```python
from build123d import *

# Parameters (mm, degrees)
F1_DEPTH  = 25.4
F0_W      = 9.8233733336
F0_H      = 1.6087094842
F2_DEPTH  = 31.75
F0_H_2    = 9.4561445239
F3_DEPTH  = 19.05
F5_DEPTH  = 4.318
F8_R      = 4.125
F9_DEPTH  = 7
F11_R     = 4.125
F7_R      = 4.125
F12_DEPTH = 15.24
F6_R      = 4.125
F10_R     = 4.125
F13_DEPTH = 15.24
F14_DEPTH = 6.35
F15_DEPTH = 6.35


with BuildPart() as f1:
    # F0 (on Front) → F1 (new body, symmetric)
    with BuildSketch(Plane.XZ):
        Polygon((38.1, 9.4561445239), (-35.3728867915, 9.4561445239), (-38.1, 7.3570762504), (-38.1, 1.6087094842), (-28.2766266664, 1.6087094842), (-28.2766266664, 0), (-28.2766266664, -9.4561445239), (28.2766266664, -9.4561445239), (28.2766266664, 0), (28.2766266664, 1.6087094842), (38.1, 1.6087094842), align=None)
    extrude(amount=F1_DEPTH, both=True)

    # F0 (on Front) → F2 (join, symmetric)
    with BuildSketch(Plane.XZ):
        with Locations((-33.1883133332, 0.8043547421)):
            Rectangle(F0_W, F0_H)
        with Locations((33.1883133332, 0.8043547421)):
            Rectangle(F0_W, F0_H)
    extrude(amount=F2_DEPTH, both=True)

    # F0 (on Front) → F3 (join, symmetric)
    with BuildSketch(Plane.XZ):
        with Locations((-33.1883133332, -4.728072262)):
            Rectangle(F0_W, F0_H_2)
        with Locations((33.1883133332, -4.728072262)):
            Rectangle(F0_W, F0_H_2)
    extrude(amount=F3_DEPTH, both=True)

    # F4 (on face) → F5 (join)
    with BuildSketch(Plane(origin=(-38.1, 0, 0), x_dir=(0, -1, 0), z_dir=(-1, 0, 0))):
        Polygon((-19.05, 0), (19.05, 0), (25.4, 0), (25.4, 1.6087094842), (25.4, 7.3570762504), (-25.4, 7.3570762504), (-25.4, 1.6087094842), (-25.4, 0), align=None)
    extrude(amount=F5_DEPTH)

    # F8 (on face) → F9 (join)
    with BuildSketch(Plane.XY.offset(9.4561445239)):
        Circle(F8_R)
    extrude(amount=F9_DEPTH)

    # F11 (on face) + F7 (on face) → F12 (join)
    with BuildSketch(Plane(origin=(0, 19.05, 0), x_dir=(-1, 0, 0), z_dir=(0, 1, 0))):
        with Locations((-33.721, -5.0771445239)):
            Circle(F11_R)
    with BuildSketch(Plane(origin=(0, 19.05, 0), x_dir=(-1, 0, 0), z_dir=(0, 1, 0))):
        with Locations((33.721, -5.0771445239)):
            Circle(F7_R)
    extrude(amount=F12_DEPTH)

    # F6 (on face) + F10 (on face) → F13 (join)
    with BuildSketch(Plane.XZ.offset(19.05)):
        with Locations((-33.721, -5.0771445239)):
            Circle(F6_R)
    with BuildSketch(Plane.XZ.offset(19.05)):
        with Locations((33.721, -5.0771445239)):
            Circle(F10_R)
    extrude(amount=F13_DEPTH)

    # F14 (add): faces of the model
    f14_faces = [f1.faces().sort_by_distance(p)[0] for p in [
        (-33.1883133332, -19.05, -0.1363515064),
        (33.1883133332, -19.05, -9.3197930175),
    ]]
    extrude(f14_faces, amount=F14_DEPTH)

    # F15 (add): faces of the model
    f15_faces = [f1.faces().sort_by_distance(p)[0] for p in [
        (33.1883133332, 19.05, -9.3197930175),
        (-33.1883133332, 19.05, -0.1363515064),
    ]]
    extrude(f15_faces, amount=F15_DEPTH)


solid = f1.part
```
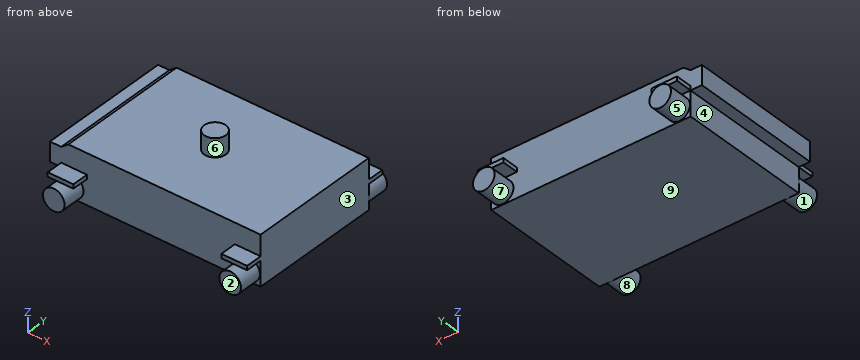
Verification items for the finished model (mm, model axes). Face numbers are marked on the shaded views. A direction names the side the tool comes from. Round coordinates to 2 decimals unless told otherwise and drop trailing zeros. Loops run counter-clockwise (first coordinate to the right, second up) from the corner with the lowest first, then second, coordinate; pieces in that order, holes last. Notation, with made-up numbers: (50, 86.5) -> (105, 86.5) arc R12 ccw to (105, 109.5) -> close; hole circle Ø3 at (43.25, 32). An arc over 180 degrees is marked (long way). Answer as a JSON object with one key per item and string values.
Q1. Section check C-C (z = -2.5). Record the boundary of the cut face in (x, y).
Data:
{"outline": "(-38.1, -25.4) -> (-36.94, -25.4) -> (-36.94, -34.29) -> (-30.5, -34.29) -> (-30.5, -25.4) -> (30.5, -25.4) -> (30.5, -34.29) -> (36.94, -34.29) -> (36.94, -25.4) -> (38.1, -25.4) -> (38.1, 25.4) -> (36.94, 25.4) -> (36.94, 34.29) -> (30.5, 34.29) -> (30.5, 25.4) -> (-30.5, 25.4) -> (-30.5, 34.29) -> (-36.94, 34.29) -> (-36.94, 25.4) -> (-38.1, 25.4) -> close"}
Q2. Scan lines: line 1 (Z direction, x = -24, y = -10.5); line 2 (Y direction, x = 32, z = 0.5); line 3 (Y direction, x = 8.5, z = -4.75). Record each from-to range of solid material in increasing order. Write a range as from..to.
Data:
{"line 1": "z = -9.46..9.46", "line 2": "y = -31.75..31.75", "line 3": "y = -25.4..25.4"}
Q3. Section check D-D (x = 9.5). Record the boundary of the cut face in (y, z), then the cut area to 3 significant figures.
Data:
{"outline": "(-25.4, -9.46) -> (25.4, -9.46) -> (25.4, 9.46) -> (-25.4, 9.46) -> close", "area": "961 mm2"}
Q4. Access from +Z, -Z, +X, -X, +Y, -Y to the whole of each face (thin tool, end or side, straight path). Record for the marked faces 1, 2, 3, 4 and 5.
Data:
{"face 1": "-Y", "face 2": "+Z, -Z, +X, -X, -Y", "face 3": "+Z, -Z, +X, +Y, -Y", "face 4": "-Z, -X, +Y, -Y", "face 5": "+Y"}
Q5. Section check A-A (x = 0). Record the boundary of the cut face in (y, z) (3 decimals), then the cut area to 3 significant figures.
Data:
{"outline": "(-25.4, -9.456) -> (25.4, -9.456) -> (25.4, 9.456) -> (4.125, 9.456) -> (4.125, 16.456) -> (-4.125, 16.456) -> (-4.125, 9.456) -> (-25.4, 9.456) -> close", "area": "1,020 mm2"}
Q6. Section check B-B (y = 15.5). Record the boundary of the cut face in (x, z).
Data:
{"outline": "(-42.42, 0) -> (-38.1, 0) -> (-38.1, -9.46) -> (38.1, -9.46) -> (38.1, 9.46) -> (-35.37, 9.46) -> (-38.1, 7.36) -> (-42.42, 7.36) -> close"}
Q7. Go/stop test with flat-tipped pins: P1, Ø3, axis at x = 28.5, z = 9.5, coming from the +Y side; P2, Ø7, axis at x = -33, y = 28.5, coming from the +Z side; P3, Ø0.8, axis at y = 27, z = 0.5, coming from the -X side. Record where each tip stops, or that it passes through.
Data:
{"P1": "stops at y = 25.4", "P2": "stops at z = 9.46", "P3": "stops at x = -38.1"}
Q8. Draft check along Z on the marked faces 6, 7, 8 and 9. Enter one of: pulls with the +Z half, pulls with the -Z half, needs draft (parallel to the pull), parting line crosses it, or undercut.
Data:
{"face 6": "needs draft", "face 7": "undercut", "face 8": "undercut", "face 9": "pulls with the -Z half"}
